from build123d import *

# Parameters (mm, degrees)
SKETCH1_W               = 3
SKETCH1_H               = 3
BOSS_EXTRUDE1_DEPTH     = 13.9
SKETCH2_W               = 3
SKETCH2_H               = 3
BOSS_EXTRUDE2_DEPTH     = 2
BOSS_EXTRUDE2_DRAFT     = -30
MIRROR1_COPY_1_SKETCH_W = 3
MIRROR1_COPY_1_SKETCH_H = 3
MIRROR1_COPY_1_DEPTH    = 2
MIRROR1_COPY_1_DRAFT    = -30
BOSS_EXTRUDE3_DEPTH     = 1.5
CUT_EXTRUDE1_REACH      = 20.085


with BuildPart() as part:
    # Sketch1 → Boss-Extrude1 (new body)
    with BuildSketch(Plane.XY):
        Rectangle(SKETCH1_W, SKETCH1_H)
    extrude(amount=BOSS_EXTRUDE1_DEPTH)


with BuildPart() as boss_extrude2_tool:
    # Sketch2 → Boss-Extrude2 (with draft: the straight prism first)
    with BuildSketch(Plane.XY.offset(13.9)):
        Rectangle(SKETCH2_W, SKETCH2_H)
    extrude(amount=BOSS_EXTRUDE2_DEPTH)
    # Boss-Extrude2: the draft: its side faces are tilted about the plane it starts from
    boss_extrude2_sides = [boss_extrude2_tool.faces().sort_by_distance(p)[0] for p in [
        (1.5, 0, 14.9),
        (0, 1.5, 14.9),
        (-1.5, 0, 14.9),
        (0, -1.5, 14.9),
    ]]
    draft(boss_extrude2_sides, Plane.XY.offset(13.9), BOSS_EXTRUDE2_DRAFT)


with BuildPart() as part_1:
    add(part.part)

    # Boss-Extrude2: add boss_extrude2_tool
    add(boss_extrude2_tool.part)


with BuildPart() as mirror1_copy_1_tool:
    # Mirror1 copy 1 sketch → Mirror1 copy 1 (with draft: the straight prism first)
    with BuildSketch(Plane(origin=(0, 0, 0), x_dir=(1, 0, 0), z_dir=(0, 0, -1))):
        Rectangle(MIRROR1_COPY_1_SKETCH_W, MIRROR1_COPY_1_SKETCH_H)
    extrude(amount=MIRROR1_COPY_1_DEPTH)
    # Mirror1 copy 1: the draft: its side faces are tilted about the plane it starts from
    mirror1_copy_1_sides = [mirror1_copy_1_tool.faces().sort_by_distance(p)[0] for p in [
        (1.5, 0, -1),
        (0, 1.5, -1),
        (-1.5, 0, -1),
        (0, -1.5, -1),
    ]]
    draft(mirror1_copy_1_sides, Plane(origin=(0, 0, 0), x_dir=(1, 0, 0), z_dir=(0, 0, -1)), MIRROR1_COPY_1_DRAFT)


with BuildPart() as part_2:
    add(part_1.part)

    # Mirror1 copy 1: add mirror1_copy_1_tool
    add(mirror1_copy_1_tool.part)

    # Sketch3 → Boss-Extrude3 (add)
    with BuildSketch(Plane.XY.offset(15.9)):
        Polygon((0, 0.866025404), (-1, -0.866025404), (1, -0.866025404), align=None)
    boss_extrude3 = extrude(amount=BOSS_EXTRUDE3_DEPTH)

    # Mirror2: Boss-Extrude3 across plane
    add(boss_extrude3.mirror(Plane.XY.offset(6.95)))

    # Sketch7 → Cut-Extrude1 (cut, up to next)
    with BuildSketch(Plane(origin=(1.5, 0, 0), x_dir=(0, 0, -1), z_dir=(1, 0, 0)), mode=Mode.PRIVATE) as cut_extrude1_sk1:
        with BuildLine():
            Line((-12.9, 0.25), (-11.4, 0.25))
            ThreePointArc((-11.4, 0.25), (-11.15, 0), (-11.4, -0.25))
            Line((-11.4, -0.25), (-12.9, -0.25))
            ThreePointArc((-12.9, -0.25), (-13.15, 0), (-12.9, 0.25))
        make_face()
    cut_extrude1_tool1 = extrude(cut_extrude1_sk1.sketch, amount=-CUT_EXTRUDE1_REACH, mode=Mode.PRIVATE) & part_2.part
    # Sketch7 → Cut-Extrude1 (cut, up to next)
    with BuildSketch(Plane(origin=(1.5, 0, 0), x_dir=(0, 0, -1), z_dir=(1, 0, 0)), mode=Mode.PRIVATE) as cut_extrude1_sk2:
        with BuildLine():
            Line((-10.4, 0.25), (-8.9, 0.25))
            ThreePointArc((-8.9, 0.25), (-8.65, 0), (-8.9, -0.25))
            Line((-8.9, -0.25), (-10.4, -0.25))
            ThreePointArc((-10.4, -0.25), (-10.65, 0), (-10.4, 0.25))
        make_face()
    cut_extrude1_tool2 = extrude(cut_extrude1_sk2.sketch, amount=-CUT_EXTRUDE1_REACH, mode=Mode.PRIVATE) & part_2.part
    # Sketch7 → Cut-Extrude1 (cut, up to next)
    with BuildSketch(Plane(origin=(1.5, 0, 0), x_dir=(0, 0, -1), z_dir=(1, 0, 0)), mode=Mode.PRIVATE) as cut_extrude1_sk3:
        with BuildLine():
            Line((-7.9, 0.25), (-6.4, 0.25))
            ThreePointArc((-6.4, 0.25), (-6.15, 0), (-6.4, -0.25))
            Line((-6.4, -0.25), (-7.9, -0.25))
            ThreePointArc((-7.9, -0.25), (-8.15, 0), (-7.9, 0.25))
        make_face()
    cut_extrude1_tool3 = extrude(cut_extrude1_sk3.sketch, amount=-CUT_EXTRUDE1_REACH, mode=Mode.PRIVATE) & part_2.part
    # Sketch7 → Cut-Extrude1 (cut, up to next)
    with BuildSketch(Plane(origin=(1.5, 0, 0), x_dir=(0, 0, -1), z_dir=(1, 0, 0)), mode=Mode.PRIVATE) as cut_extrude1_sk4:
        with BuildLine():
            Line((-5.4, 0.25), (-3.9, 0.25))
            ThreePointArc((-3.9, 0.25), (-3.65, 0), (-3.9, -0.25))
            Line((-3.9, -0.25), (-5.4, -0.25))
            ThreePointArc((-5.4, -0.25), (-5.65, 0), (-5.4, 0.25))
        make_face()
    cut_extrude1_tool4 = extrude(cut_extrude1_sk4.sketch, amount=-CUT_EXTRUDE1_REACH, mode=Mode.PRIVATE) & part_2.part
    # Sketch7 → Cut-Extrude1 (cut, up to next)
    with BuildSketch(Plane(origin=(1.5, 0, 0), x_dir=(0, 0, -1), z_dir=(1, 0, 0)), mode=Mode.PRIVATE) as cut_extrude1_sk5:
        with BuildLine():
            Line((-2.9, 0.25), (-1.4, 0.25))
            ThreePointArc((-1.4, 0.25), (-1.15, 0), (-1.4, -0.25))
            Line((-1.4, -0.25), (-2.9, -0.25))
            ThreePointArc((-2.9, -0.25), (-3.15, 0), (-2.9, 0.25))
        make_face()
    cut_extrude1_tool5 = extrude(cut_extrude1_sk5.sketch, amount=-CUT_EXTRUDE1_REACH, mode=Mode.PRIVATE) & part_2.part
    add(cut_extrude1_tool1.solids().sort_by_distance((1.5, 0, 12.15))[0], mode=Mode.SUBTRACT)
    add(cut_extrude1_tool2.solids().sort_by_distance((1.5, 0, 9.65))[0], mode=Mode.SUBTRACT)
    add(cut_extrude1_tool3.solids().sort_by_distance((1.5, 0, 7.15))[0], mode=Mode.SUBTRACT)
    add(cut_extrude1_tool4.solids().sort_by_distance((1.5, 0, 4.65))[0], mode=Mode.SUBTRACT)
    add(cut_extrude1_tool5.solids().sort_by_distance((1.5, 0, 2.15))[0], mode=Mode.SUBTRACT)


solid = part_2.part
Input: part model. Units: mm. Frame: model coordinates. A direction names the side the tool comes from. Give positions to 0.01 mm unless a question says otherwise; leave off trailing zeros. Loops run counter-clockwise (first coordinate to the right, second up) from the corner with the lowest first, then second, coordinate; pieces in that order, holes last. Notation, with made-up numbers: M -19.5,-23.5 L 13.5,-23.5 A26 ccw 13.5,11.5 Z; hole C -2.5,66 d1. An arc over 180 degrees is marked long. Use one line per item in the form item = value.
1. First-contact query: pin 1 (0.8 mm diameter, centred on x = 0.5, z = 2, fed in from -Y); pin 2 (2 mm diameter, centred on y = 1.5, z = 2, fed in from -X); pin 3 (0.5 mm diameter, centred on x = 0, z = 2.5, fed in from +Y); pin 4 (1.6 mm diameter, centred on x = 1, y = 0.5, fed in from +Z). Flat tips, straight axial feed; report the tip coordinate or a pass-through.
Numbers:
pin_1 = -1.5
pin_2 = -1.5
pin_3 = 1.5
pin_4 = 17.4
2. Pull-direction query (Y, two-part tool) for faces 1 (the face through (-2.07, 0.04, -0.99)), 2 (the face through (0, 0.25, 12)), 3 (the face through (-0.04, -2.07, 14.89)), 4 (the face through (0, 0.25, 10)); classes: released by +Y, released by -Y, zero draft, split by the parting line, or undercut.
Numbers:
face_1 = zero draft
face_2 = undercut
face_3 = released by -Y
face_4 = undercut
3. Section query C-C, the plane y = 0. Count the separate pieces of the cut face and the enclosed holes in it, and give its area (3 significant figures).
Numbers:
separate_pieces = 6
enclosed_holes = 0
area = 31.3 mm²
4. Line query: L1, parallel to Z at x = 0.4, y = -0.05; L2, parallel to X at y = -0.3, z = 5.5; L3, parallel to Y at x = -0.2, z = 1.5. Output: solid intervals per line, ascending.
Numbers:
L1 = -3.5 to 1.16, 3.14 to 3.66, 5.64 to 6.16, 8.14 to 8.66, 10.64 to 11.16, 13.14 to 17.4
L2 = -1.5 to 1.5
L3 = -1.5 to -0.25, 0.25 to 1.5
5. Section query B-B, the plane y = 1.9. Return the cut outline in (x, z).
Numbers:
outline = M -2.65,-2 L 2.65,-2 L 1.9,-0.69 L -1.9,-0.69 Z; M -2.65,15.9 L -1.9,14.59 L 1.9,14.59 L 2.65,15.9 Z
6. Reachability of faces 5 (the face through (0.5, 0, -2.7)), 6 (the face through (-0.04, 2.07, 14.89)), 7 (the face through (-0.04, -2.07, -0.99)), 8 (the face through (0, 0.25, 7)), 9 (the face through (-0.5, 0, 16.6)) from +Z, -Z, +X, -X, +Y, -Y: full face, straight path, thin tool, end or side. Return the list, or none.
Numbers:
face_5 = -Z, +X, +Y
face_6 = +X, -X, +Y
face_7 = +X, -X, -Y
face_8 = +X, -X
face_9 = +Z, -X, +Y
7. Section query A-A, the plane z = 7.25. Return the cut outline in (x, y), and give its area (3 significant figures).
Numbers:
outline = M -1.5,-1.5 L 1.5,-1.5 L 1.5,-0.25 L -1.5,-0.25 Z; M -1.5,0.25 L 1.5,0.25 L 1.5,1.5 L -1.5,1.5 Z
area = 7.50 mm²
